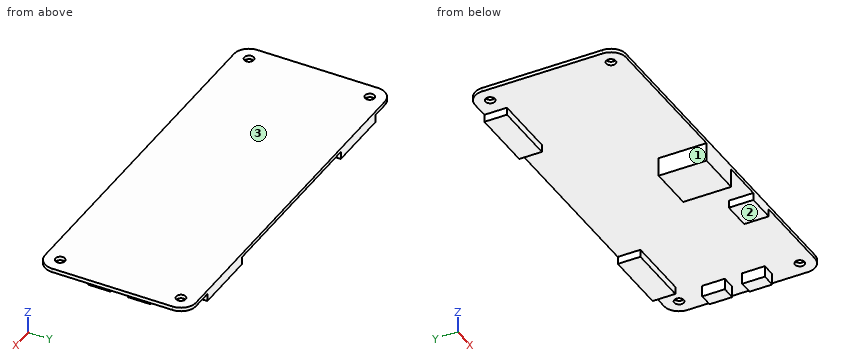
Solid Edge part; units mm, degrees
sketch "Sketch1" plane through (0, 0, 0) normal (0, 0, 1) x (1, 0, 0)
  line L0 (-50, -20) -> (50, -20)
  line L1 (50, -20) -> (50, 20)
  line L2 (50, 20) -> (-50, 20)
  line L3 (-50, 20) -> (-50, -20)
  circle A0 centre (-46, -16) radius 1.25
  circle A1 centre (-46, 16) radius 1.25
  circle A2 centre (46, 16) radius 1.25
  circle A3 centre (46, -16) radius 1.25
extrude "Protrusion1" add sketch "Sketch1" along normal blind 1
fillet "Round_1" radius 4 4 edges at (-50, -20, 0.5) (-50, 20, 0.5) (50, -20, 0.5) (50, 20, 0.5)
sketch "Sketch2" plane through (0, 0, 0) normal (0, 0, 1) x (1, 0, 0)
  line L0 (-24.5, 14) -> (-24.5, 20)
  line L1 (-24.5, 20) -> (-41.5, 20)
  line L2 (-41.5, 20) -> (-41.5, 14)
  line L3 (-41.5, 14) -> (-24.5, 14)
  line L4 (23.5, 20) -> (23.5, 14)
  line L5 (23.5, 14) -> (40.5, 14)
  line L6 (40.5, 14) -> (40.5, 20)
  line L7 (40.5, 20) -> (23.5, 20)
extrude "ExtrudedProtrusion_2" add sketch "Sketch2" against normal blind 2
sketch "Sketch3" plane through (0, 0, 0) normal (0, 0, 1) x (1, 0, 0)
  line L0 (5.2, -7.3029) -> (5.2, -20)
  line L1 (5.2, -20) -> (-6.8, -20)
  line L2 (-6.8, -20) -> (-6.8, -7.3029)
  line L3 (-6.8, -7.3029) -> (5.2, -7.3029)
extrude "ExtrudedProtrusion_3" add sketch "Sketch3" against normal blind 5
sketch "Sketch4" plane through (0, 0, 0) normal (0, 0, 1) x (1, 0, 0)
  line L0 (23.5, -20) -> (23.5, -13.5)
  line L1 (23.5, -13.5) -> (16, -13.5)
  line L2 (16, -13.5) -> (16, -20)
  line L3 (16, -20) -> (23.5, -20)
extrude "ExtrudedProtrusion_4" add sketch "Sketch4" against normal blind 2
sketch "Sketch5" plane through (0, 0, 0) normal (0, 0, 1) x (1, 0, 0)
  line L0 (46.72, -2.3) -> (46.72, -8.3)
  line L1 (46.72, -8.3) -> (43.12, -8.3)
  line L2 (43.12, -8.3) -> (43.12, -2.3)
  line L3 (43.12, -2.3) -> (46.72, -2.3)
  line L4 (46.72, 8.3) -> (46.72, 2.3)
  line L5 (46.72, 2.3) -> (43.12, 2.3)
  line L6 (43.12, 2.3) -> (43.12, 8.3)
  line L7 (43.12, 8.3) -> (46.72, 8.3)
extrude "ExtrudedProtrusion_5" add sketch "Sketch5" against normal blind 3
Geometry check sheet. Reference: the model listing, model coordinates, mm. Face numbers are marked on the shaded views. A direction names the side the tool comes from. Round coordinates to 2 decimals unless told otherwise and drop trailing zeros. Write each loop counter-clockwise with the first axis right and the second up, starting at its lowest first coordinate (ties: lowest second). Pieces come first, ordered by that corner, then holes. Notation, with made-up numbers: (-3.75, 30.25) - (21.25, 30.25) arc R18 cw to (21.25, 48.25) - close; hole circle Ø9 at (14, 1.5). An arc over 180 degrees is marked (long way). Write each question's results on one line, items separated by ' | '.
(1) Set-up check for the marked faces 1, 2 and 3: record each of +Z, -Z, +X, -X, +Y, -Y from which the full face is reachable in a straight line by a thin tool's end or side.
Computed:
face 1: -Z, -X, +Y, -Y | face 2: -Z, +X, +Y, -Y | face 3: +Z, +X, -X, +Y, -Y
(2) Sectioned sample at B-B, the plane x = -3. Enter the section's corners in (y, z).
Computed:
outline: (-20, -5) - (-7.3, -5) - (-7.3, 0) - (20, 0) - (20, 1) - (-20, 1) - close
(3) Depth check by flat-ended pin: pin 1 Ø0.6 at (y, z) = (18.5, -1) entering from -X; pin 2 Ø1.5 at (x, z) = (-2, -3) entering from +Y; pin 3 Ø0.6 at (y, z) = (17.5, -0.5) entering from +X. Enter the tip coordinate at first touch or a pass-through.
Computed:
pin 1: stops at x = -41.5 | pin 2: stops at y = -7.3 | pin 3: stops at x = 40.5
(4) Sectioned sample at A-A, the plane z = -1.05. Enter the section's corners in (x, y).
Computed:
outline: (-41.5, 14) - (-24.5, 14) - (-24.5, 20) - (-41.5, 20) - close; (-6.8, -20) - (5.2, -20) - (5.2, -7.3) - (-6.8, -7.3) - close; (16, -20) - (23.5, -20) - (23.5, -13.5) - (16, -13.5) - close; (23.5, 14) - (40.5, 14) - (40.5, 20) - (23.5, 20) - close; (43.12, -8.3) - (46.72, -8.3) - (46.72, -2.3) - (43.12, -2.3) - close; (43.12, 2.3) - (46.72, 2.3) - (46.72, 8.3) - (43.12, 8.3) - close
(5) Sectioned sample at D-D, the plane x = -33. Enter the section's corners in (y, z), plus the area to 3 significant figures.
Computed:
outline: (-20, 0) - (14, 0) - (14, -2) - (20, -2) - (20, 1) - (-20, 1) - close | area: 52.0 mm^2
(6) Sectioned sample at C-C, the plane y = 12. Enter the section's corners in (x, z), plus the area to 3 significant figures.
Computed:
outline: (-50, 0) - (50, 0) - (50, 1) - (-50, 1) - close | area: 100 mm^2
(7) Thickness scan on probe 1 along Y at (x, z) = (46, 0.6); probe 2 along X at (y, z) = (-4, -2.6); probe 3 along Z at (x, y) = (20.5, -16). Record the ranges inside material, lowest first. Write a range as from..to.
Computed:
probe 1: y = -20..-17.25, -14.75..14.75, 17.25..20 | probe 2: x = 43.12..46.72 | probe 3: z = -2..1
